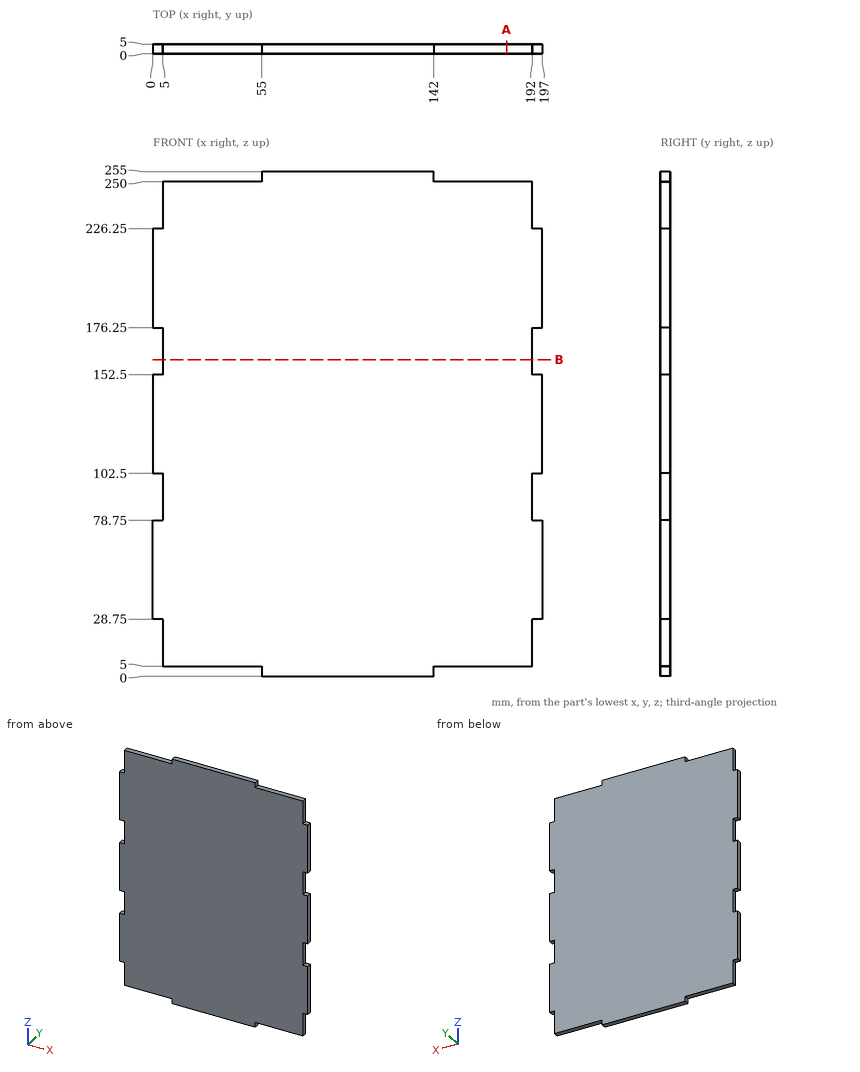
Drawing for the job (mm, zero at the part's lowest x, y, z). Give positions to 0.01 mm unless a question says otherwise; leave off trailing zeros. Order: outer loops, then holes, each group sorted by start corner. A loop starts at its lowest first (then second) coordinate and runs counter-clockwise, first axis right, second up. Notation, with made-up numbers: (46.5, 63.5) -> (50.5, 63.5) arc R15 ccw to (50.5, 82.5) -> close; hole circle Ø10 at (22, 10). An arc over 180 degrees is marked (long way). Use one line per item in the form item = value.
(1) Saw through at A-A (x = 179). Write the cut outline in (y, z), then the cut area to 4 significant figures.
Solution:
outline = (0, 5) -> (5, 5) -> (5, 250) -> (0, 250) -> close
area = 1,225 mm²
(2) Saw through at B-B (z = 160). Write the cut outline in (x, y), then the cut area to 3 significant figures.
Solution:
outline = (5, 0) -> (192, 0) -> (192, 5) -> (5, 5) -> close
area = 935 mm²
(3) Drill centre lines: line 1 (X direction, y = 1.05, z = 240); line 2 (Z direction, x = 12.5, y = 2.5). Where is each one in solid material? Low to high. Write a range as from..to.
Solution:
line_1 = 5..192
line_2 = 5..250
(4) Flat gauge pins, fed straight in: P1, Ø2.5, axis at x = 2.5, y = 3.5, coming from the -Z side; P2, Ø2.5, axis at x = 3.5, y = 2, coming from the +Z side; P3, Ø2.5, axis at x = 157.5, y = 2, coming from the -Z side. Where does each tip first touch, or does it go through?
Solution:
P1 = 28.75
P2 = 226.25
P3 = 5
